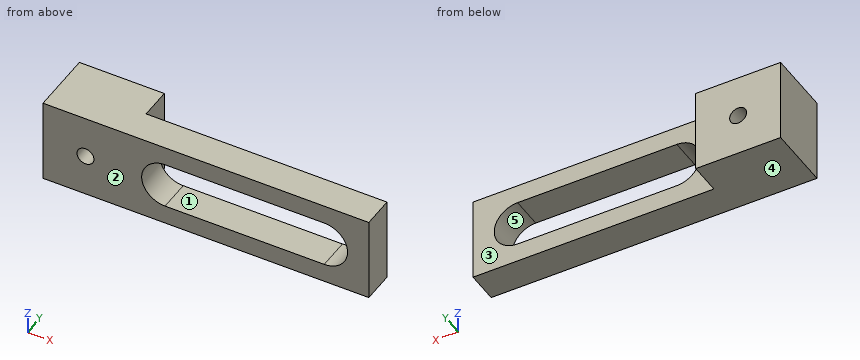
from build123d import *

# Parameters (mm, degrees)
SKETCH1_W           = 30.7
SKETCH1_H           = 8
BOSS_EXTRUDE1_DEPTH = 3
SKETCH2_W           = 8
SKETCH2_H           = 8
BOSS_EXTRUDE2_DEPTH = 3
CUT_EXTRUDE1_REACH  = 22.51
SKETCH3_R           = 0.8


with BuildPart() as part:
    # Sketch1 → Boss-Extrude1 (new body)
    with BuildSketch(Plane(origin=(0, 0, 0), x_dir=(1, 0, 0), z_dir=(0, 1, 0))):
        with Locations((3.85, 0)):
            Rectangle(SKETCH1_W, SKETCH1_H)
        with BuildLine():
            Line((0, 2.2), (15, 2.2))
            ThreePointArc((15, 2.2), (17.2, 0), (15, -2.2))
            Line((15, -2.2), (0, -2.2))
            ThreePointArc((0, -2.2), (-2.2, 0), (0, 2.2))
        make_face(mode=Mode.SUBTRACT)
    extrude(amount=BOSS_EXTRUDE1_DEPTH)

    # Sketch2 → Boss-Extrude2 (add)
    with BuildSketch(Plane(origin=(0, 3, 0), x_dir=(1, 0, 0), z_dir=(0, 1, 0))):
        with Locations((-7.5, 0)):
            Rectangle(SKETCH2_W, SKETCH2_H)
    extrude(amount=BOSS_EXTRUDE2_DEPTH)

    # Sketch3 → Cut-Extrude1 (cut, up to next)
    with BuildSketch(Plane(origin=(0, 6, 0), x_dir=(1, 0, 0), z_dir=(0, 1, 0)), mode=Mode.PRIVATE) as cut_extrude1_sk1:
        with Locations(Location((-7.5, 0, 0), (0, 0, 270))):
            Circle(SKETCH3_R)
    cut_extrude1_tool1 = extrude(cut_extrude1_sk1.sketch, amount=-CUT_EXTRUDE1_REACH, mode=Mode.PRIVATE) & part.part
    add(cut_extrude1_tool1.solids().sort_by_distance((-7.5, 6, 0))[0], mode=Mode.SUBTRACT)


solid = part.part
For this review, take the finished solid that the model builds, in its own axes (mm). Face numbers are marked on the shaded views. A direction names the side the tool comes from. Round coordinates to 2 decimals unless told otherwise and drop trailing zeros. Order: outer loops, then holes, each group sorted by start corner. A loop starts at its lowest first (then second) coordinate and runs counter-clockwise, first axis right, second up. Notation, with made-up numbers: M 70.25,-27 L 106.25,-27 A18 ccw 106.25,-11 Z; hole C 67.5,73.5 d2. An arc over 180 degrees is marked long. Write each question's results on one line, items separated by ' | '. Start each with the question number.
1. Add section C-C (y = 2.2). State the section outline as (x, z) points.
2. Add section D-D (x = 0.5). State the section outline as (y, z) points.
3. Tool access review of the marked faces 1 and 2: name each direction out of +Z, -Z, +X, -X, +Y, -Y from which nothing blocks a thin tool from reaching the whole face with its end or side.
4. Add section A-A (x = -7.5). State the section outline as (y, z) points.
5. Clearance check with flat-ended pins moving along their axes: pin 1 Ø4 at (x, z) = (13, 1) entering from +Y; pin 2 Ø3.5 at (y, z) = (5, 0) entering from +X. State where each tip first meets the part, or that it passes through.
6. Draft analysis for pull direction Z (two halves, no side actions). For the marked faces 3, 4 and 5, state which applies: pulls with the +Z half, pulls with the -Z half, needs draft (parallel to the pull), parting line crosses it, or undercut.
7. To check wall thickness, follow L1, parallel to X at y = 1.45, z = 0; L2, parallel to X at y = 4.85, z = 0; L3, parallel to Z at x = 3, y = 2. State the ranges of each line that lie inside material, in increasing order. Write a range as [from, to].
8. Add section B-B (z = 0). State the section outline as (x, y) points.
Output values:
1) outline: M -11.5,-4 L 19.2,-4 L 19.2,4 L -11.5,4 Z; hole C -7.5,0 d1.6; hole M 0,-2.2 L 15,-2.2 A2.2 ccw 15,2.2 L 0,2.2 A2.2 ccw Z
2) outline: M 0,-4 L 3,-4 L 3,-2.2 L 0,-2.2 Z; M 0,2.2 L 3,2.2 L 3,4 L 0,4 Z
3) face 1: +Y, -Y | face 2: +Z, -Z, +X, -X, -Y
4) outline: M 0,-4 L 6,-4 L 6,-0.8 L 0,-0.8 Z; M 0,0.8 L 6,0.8 L 6,4 L 0,4 Z
5) pin 1: y = 3 | pin 2: x = -3.5
6) face 3: needs draft | face 4: pulls with the -Z half | face 5: undercut
7) L1: [-11.5, -8.3], [-6.7, -2.2], [17.2, 19.2] | L2: [-11.5, -8.3], [-6.7, -3.5] | L3: [-4, -2.2], [2.2, 4]
8) outline: M -11.5,0 L -8.3,0 L -8.3,6 L -11.5,6 Z; M -6.7,0 L -2.2,0 L -2.2,3 L -3.5,3 L -3.5,6 L -6.7,6 Z; M 17.2,0 L 19.2,0 L 19.2,3 L 17.2,3 Z
